The model under review builds one solid part; all positions refer to its coordinate system, in mm. Face numbers are marked on the shaded views. Coordinates: 2 decimals unless noted, no trailing zeros. Order: outer loops, then holes, each group sorted by start corner. A loop starts at its lowest first (then second) coordinate and runs counter-clockwise, first axis right, second up. Notation, with made-up numbers: M -20.5,83 L -14.5,83 A17 cw -14.5,110 Z; hole C 44.25,-7 d11. An arc over 180 degrees is marked long. Write each question's results on one line, items separated by ' | '.
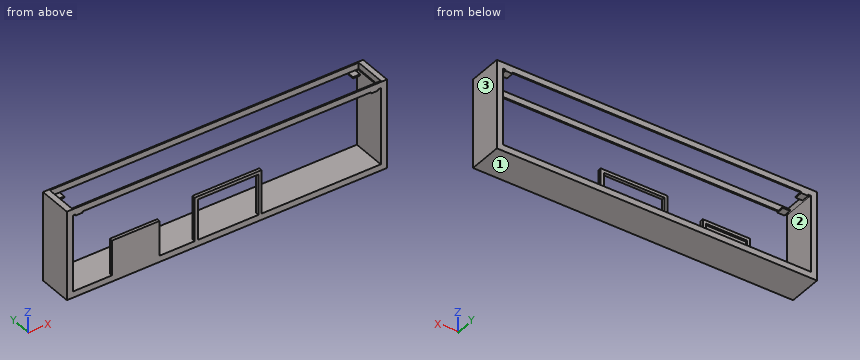
from build123d import *

# Parameters (mm, degrees)
SKETCH2_W               = 512.8
SKETCH2_H               = 142.48
SKETCH2_W_2             = 492.8
SKETCH2_H_2             = 122.48
EXTRUDE_THIN1_DEPTH     = 54
SKETCH3_W               = 495
SKETCH3_H               = 50
CUT_EXTRUDE1_DEPTH      = 10
SKETCH4_W               = 11.198987657
SKETCH4_H               = 12.828632872
BOSS_EXTRUDE1_DEPTH     = 2
MIRROR3_COPY_1_SKETCH_W = 11.198987657
MIRROR3_COPY_1_SKETCH_H = 12.828632872
MIRROR3_COPY_1_DEPTH    = 2
MIRROR3_COPY_2_SKETCH_W = 11.198987657
MIRROR3_COPY_2_SKETCH_H = 12.828632872
MIRROR3_COPY_2_DEPTH    = 2
SKETCH5_W               = 5
SKETCH5_H               = 5
BOSS_EXTRUDE2_DEPTH     = 70
SKETCH7_W               = 5
SKETCH7_H               = 5
BOSS_EXTRUDE3_DEPTH     = 102
SKETCH8_W               = 5
SKETCH8_H               = 5
BOSS_EXTRUDE4_DEPTH     = 65
SKETCH9_W               = 5
SKETCH9_H               = 5
BOSS_EXTRUDE5_DEPTH     = 56
SKETCH10_W              = 5
SKETCH10_H              = 5
BOSS_EXTRUDE6_DEPTH     = 71
SKETCH11_W              = 5
SKETCH11_H              = 5
BOSS_EXTRUDE7_DEPTH     = 51
SKETCH14_W              = 51
SKETCH14_H              = 2
BOSS_EXTRUDE8_DEPTH     = 66


with BuildPart() as part:
    # Sketch2 → Extrude-Thin1 (new body)
    with BuildSketch(Plane(origin=(0, 0, 0), x_dir=(1, 0, 0), z_dir=(0, 1, 0))):
        with Locations((0, 0.16)):
            Rectangle(SKETCH2_W, SKETCH2_H)
        with Locations((0, 0.16)):
            Rectangle(SKETCH2_W_2, SKETCH2_H_2, mode=Mode.SUBTRACT)
    extrude(amount=EXTRUDE_THIN1_DEPTH)

    # Sketch3 → Cut-Extrude1 (cut)
    with BuildSketch(Plane.XY.offset(71.08)):
        with Locations((0.567740689, 27.1414334)):
            Rectangle(SKETCH3_W, SKETCH3_H)
    extrude(amount=-CUT_EXTRUDE1_DEPTH, mode=Mode.SUBTRACT)

    # Sketch4 → Boss-Extrude1 (add)
    with BuildSketch(Plane(origin=(0, 0, 61.08), x_dir=(-1, 0, 0), z_dir=(0, 0, -1))):
        with Locations((236.763190304, 47.585683564)):
            Rectangle(SKETCH4_W, SKETCH4_H)
    boss_extrude1 = extrude(amount=BOSS_EXTRUDE1_DEPTH)

    # Mirror1: Boss-Extrude1 across plane
    add(boss_extrude1.mirror(Plane(origin=(0, 0, 0), x_dir=(0, 0, 1), z_dir=(1, 0, 0))))

    # Mirror2: Boss-Extrude1 across plane
    add(boss_extrude1.mirror(Plane.ZX.offset(27)))

    # Mirror3 copy 1 sketch → Mirror3 copy 1 (add)
    with BuildSketch(Plane(origin=(0, 54, 61.08), x_dir=(1, 0, 0), z_dir=(0, 0, -1))):
        with Locations((236.763190304, 47.585683564)):
            Rectangle(MIRROR3_COPY_1_SKETCH_W, MIRROR3_COPY_1_SKETCH_H)
    extrude(amount=MIRROR3_COPY_1_DEPTH)

    # Mirror3 copy 2 sketch → Mirror3 copy 2 (add)
    with BuildSketch(Plane(origin=(0, 54, 61.08), x_dir=(-1, 0, 0), z_dir=(0, 0, -1))):
        with Locations((236.763190304, -47.585683564)):
            Rectangle(MIRROR3_COPY_2_SKETCH_W, MIRROR3_COPY_2_SKETCH_H)
    extrude(amount=MIRROR3_COPY_2_DEPTH)

    # Sketch5 → Boss-Extrude2 (add)
    with BuildSketch(Plane.XY.offset(-61.4)):
        with Locations((52.881030247, 2.5)):
            Rectangle(SKETCH5_W, SKETCH5_H)
    extrude(amount=BOSS_EXTRUDE2_DEPTH)

    # Sketch7 → Boss-Extrude3 (add)
    with BuildSketch(Plane.ZY.offset(-50.381030247)):
        with Locations((6.1, 2.5)):
            Rectangle(SKETCH7_W, SKETCH7_H)
    extrude(amount=BOSS_EXTRUDE3_DEPTH)

    # Sketch8 → Boss-Extrude4 (add)
    with BuildSketch(Plane(origin=(0, 0, 3.6), x_dir=(-1, 0, 0), z_dir=(0, 0, -1))):
        with Locations((49.118969753, 2.5)):
            Rectangle(SKETCH8_W, SKETCH8_H)
    extrude(amount=BOSS_EXTRUDE4_DEPTH)

    # Sketch9 → Boss-Extrude5 (add)
    with BuildSketch(Plane.XY.offset(-61.4)):
        with Locations((-110.630872861, 2.5)):
            Rectangle(SKETCH9_W, SKETCH9_H)
    extrude(amount=BOSS_EXTRUDE5_DEPTH)

    # Sketch10 → Boss-Extrude6 (add)
    with BuildSketch(Plane.ZY.offset(113.130872861)):
        with Locations((-7.9, 2.5)):
            Rectangle(SKETCH10_W, SKETCH10_H)
    extrude(amount=BOSS_EXTRUDE6_DEPTH)

    # Sketch11 → Boss-Extrude7 (add)
    with BuildSketch(Plane(origin=(0, 0, -10.4), x_dir=(-1, 0, 0), z_dir=(0, 0, -1))):
        with Locations((181.630872861, 2.5)):
            Rectangle(SKETCH11_W, SKETCH11_H)
    extrude(amount=BOSS_EXTRUDE7_DEPTH)

    # Sketch14 → Boss-Extrude8 (add)
    with BuildSketch(Plane(origin=(-179.130872861, 0, 0), x_dir=(0, 0, -1), z_dir=(1, 0, 0))):
        with Locations((35.9, 1)):
            Rectangle(SKETCH14_W, SKETCH14_H)
    extrude(amount=BOSS_EXTRUDE8_DEPTH)


solid = part.part
1) To check wall thickness, follow line 1 along X through (y, z) = (49.5, 26.5); line 2 along Z through (x, y) = (-131, 52.5); line 3 along X through (y, z) = (48, 65). State the ranges of each line that lie inside material, in increasing order.
Solutions:
line 1: -256.4 to -246.4, 246.4 to 256.4 | line 2: -71.4 to -61.4, 61.08 to 71.08 | line 3: -256.4 to -246.93, 248.07 to 256.4
2) Take a section at C-C on x = 171. State the section outline as (y, z) points.
Solutions:
outline: M 0,-71.4 L 54,-71.4 L 54,-61.4 L 0,-61.4 Z; M 0,61.08 L 2.14,61.08 L 2.14,71.08 L 0,71.08 Z; M 52.14,61.08 L 54,61.08 L 54,71.08 L 52.14,71.08 Z
3) Take a section at D-D on x = -5.5. State the section outline as (y, z) points, plus the area to 3 significant figures.
Solutions:
outline: M 0,-71.4 L 54,-71.4 L 54,-61.4 L 0,-61.4 Z; M 0,3.6 L 5,3.6 L 5,8.6 L 0,8.6 Z; M 0,61.08 L 2.14,61.08 L 2.14,71.08 L 0,71.08 Z; M 52.14,61.08 L 54,61.08 L 54,71.08 L 52.14,71.08 Z | area: 605 mm2
4) Take a section at A-A on z = -1. State the section outline as (x, y) points, plus the area to 3 significant figures.
Solutions:
outline: M -256.4,0 L -246.4,0 L -246.4,54 L -256.4,54 Z; M -51.62,0 L -46.62,0 L -46.62,5 L -51.62,5 Z; M 50.38,0 L 55.38,0 L 55.38,5 L 50.38,5 Z; M 246.4,0 L 256.4,0 L 256.4,54 L 246.4,54 Z | area: 1,130 mm2
5) Take a section at B-B on z = 26. State the section outline as (x, y) points, plus the area to 3 significant figures.
Solutions:
outline: M -256.4,0 L -246.4,0 L -246.4,54 L -256.4,54 Z; M 246.4,0 L 256.4,0 L 256.4,54 L 246.4,54 Z | area: 1,080 mm2
6) The part is to be moulded in two halves that separate along X. For the marked faces 1, 2 and 3, say which applies: pulls with the +X half, pulls with the -X half, needs draft (parallel to the pull), parting line crosses it, or undercut.
Solutions:
face 1: needs draft | face 2: undercut | face 3: pulls with the +X half
7) For pin 1 (1 mm diameter, centred on x = -155, y = 23, fed in from +Z); pin 2 (5.5 mm diameter, centred on x = -234.5, y = 46, fed in from +Z); pin 3 (4 mm diameter, centred on x = -164, y = 2.5, fed in from +Z), all flat-tipped, find the tip position at first contact; note any pin that passes through.
Solutions:
pin 1: z = -61.4 | pin 2: z = 61.08 | pin 3: z = 71.08
